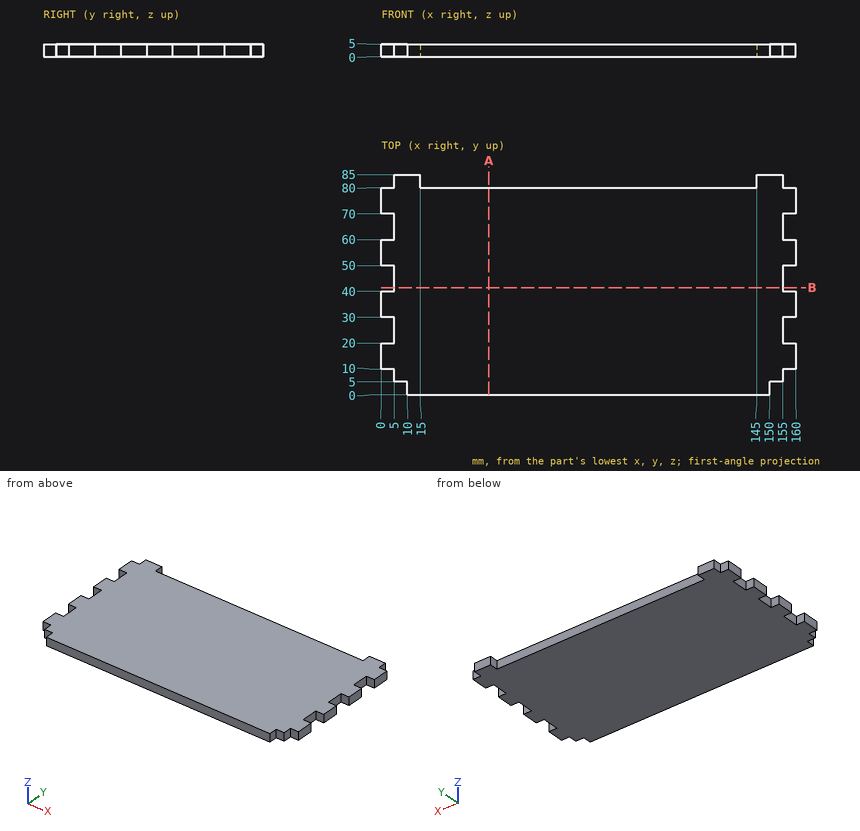
Input: dimensioned drawing with shaded views. Units: mm. Origin: part minimum x, y, z. Round coordinates to 2 decimals unless told otherwise and drop trailing zeros. Order: outer loops, then holes, each group sorted by start corner. A loop starts at its lowest first (then second) coordinate and runs counter-clockwise, first axis right, second up. Notation, with made-up numbers: (38.25, 45) -> (71.25, 45) arc R26 ccw to (71.25, 84) -> close; hole circle Ø11 at (42, -20.5). An arc over 180 degrees is marked (long way). One line per item, written item: value. Start each with the question number.
Q1. Pin query (flat end, axial travel): pin 1 (2.5 mm diameter, centred on x = 158, z = 2.5, fed in from -Y); pin 2 (2 mm diameter, centred on y = 66, z = 2, fed in from +X); pin 3 (2.5 mm diameter, centred on y = 83, z = 3.5, fed in from -X); pin 4 (1.5 mm diameter, centred on x = 69.5, y = 70.5, fed in from -Z). Return the tip coordinate at first contact, or that it passes through.
Q2. Section query B-B (y = 41.5). Return the cut outline in (x, z), plus the area to 3 significant figures.
Q3. Material intervals for probe 1 along Y at (x, z) = (153, 0.55); probe 2 along Y at (x, z) = (117, 0.2); probe 3 along X at (y, z) = (63.5, 2.7), sorted ascending.
Q4. Section query A-A (x = 41.5). Return the cut outline in (y, z), plus the area to 3 significant figures.
Findings below:
1. pin 1: y = 10
1. pin 2: x = 155
1. pin 3: x = 5
1. pin 4: z = 0
2. outline: (5, 0) -> (155, 0) -> (155, 5) -> (5, 5) -> close
2. area: 750 mm²
3. probe 1: 5 to 85
3. probe 2: 0 to 80
3. probe 3: 5 to 155
4. outline: (0, 0) -> (80, 0) -> (80, 5) -> (0, 5) -> close
4. area: 400 mm²
